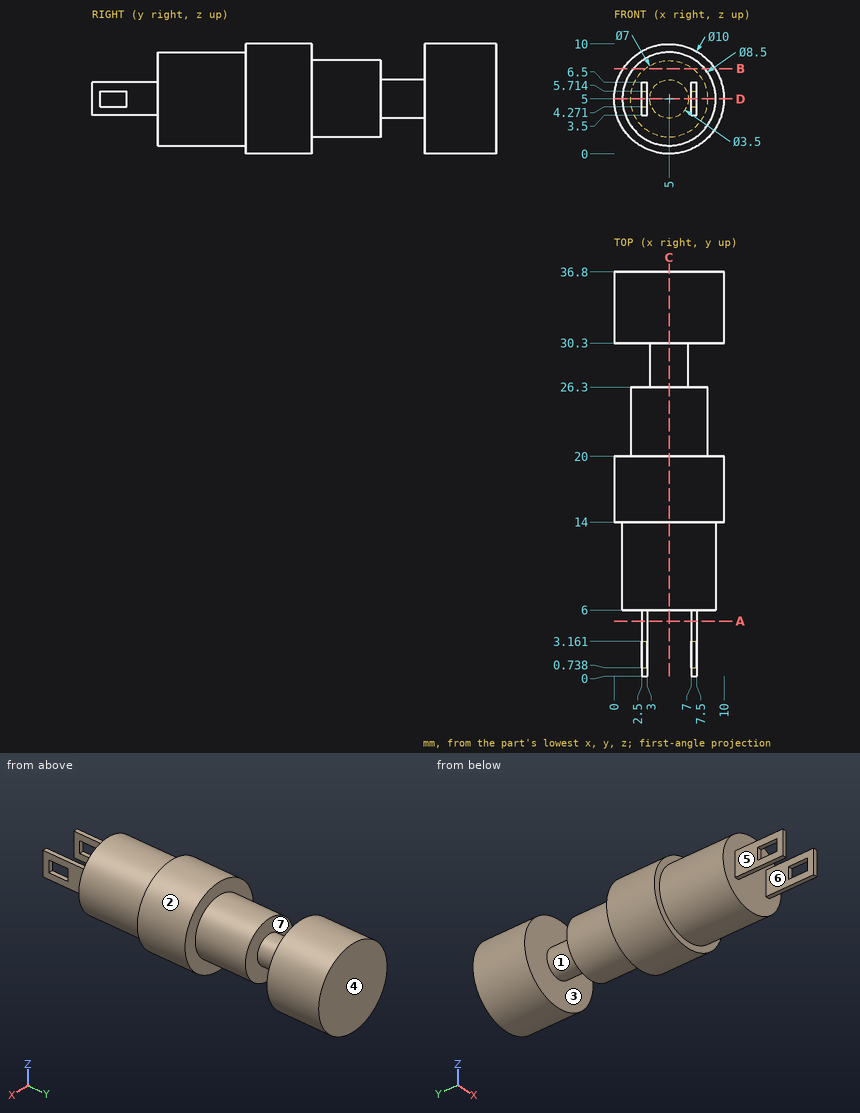
Study the drawing (mm; zero at the part's minimum x, y, z) and answer. A direction names the side the tool comes from. Give positions to 0.01 mm unless a question says otherwise; leave off trailing zeros. Order: outer loops, then holes, each group sorted by start corner. A loop starts at its lowest first (then second) coordinate and runs counter-clockwise, first axis right, second up.
1) For the marked faces 5, 6 and 7, determine the directions among +Z, -Z, +X, -X, +Y, -Y from which every point of the face is accessible in a straight line to the end or side of a thin tool.
Reported:
face 5: +Z, -Z, -X, -Y
face 6: +Z, -Z, -Y
face 7: none
2) Find section D-D on z = 5. Give the number of separate pieces and of enclosed holes in the cut face, then the cut area to 3 significant figures.
Reported:
separate pieces: 3
enclosed holes: 0
area: 255 mm2
3) Given P1, Ø3, axis at x = 6, z = 8, coming from the -Y side; P2, Ø0.9, axis at y = 2, z = 4.5, coming from the +X side; P3, Ø1, axis at x = 6, y = 19, coming from the -Z side (1 decimal), each flat-ended and moving along its own axis, determine where each tip first touches the part or whether it passes through.
Reported:
P1: stops at y = 6
P2: stops at x = 7.5
P3: stops at z = 0
4) Consider line 1 along Y through (x, z) = (5, 9); line 2 along Y through (x, z) = (6, 6.75); line 3 along Z through (x, y) = (5.25, 16). Determine where each line is inside the solid, lowest interval first.
Reported:
line 1: y = 6 to 20, 30.3 to 36.8
line 2: y = 6 to 26.3, 30.3 to 36.8
line 3: z = 0.01 to 9.99
5) Find section C-C on x = 5. Write down the section's boundary in (y, z), then the cut area to 3 significant figures.
Reported:
outline: (6, 0.75) - (14, 0.75) - (14, 0) - (20, 0) - (20, 1.5) - (26.3, 1.5) - (26.3, 3.25) - (30.3, 3.25) - (30.3, 0) - (36.8, 0) - (36.8, 10) - (30.3, 10) - (30.3, 6.75) - (26.3, 6.75) - (26.3, 8.5) - (20, 8.5) - (20, 10) - (14, 10) - (14, 9.25) - (6, 9.25) - close
area: 251 mm2
6) Find section B-B on z = 7.75. Write down the section's boundary in (x, y) (1 decimal).
Reported:
outline: (0.8, 14) - (1.8, 14) - (1.8, 6) - (8.2, 6) - (8.2, 14) - (9.2, 14) - (9.2, 20) - (7.2, 20) - (7.2, 26.3) - (2.8, 26.3) - (2.8, 20) - (0.8, 20) - close; (0.8, 30.3) - (9.2, 30.3) - (9.2, 36.8) - (0.8, 36.8) - close
7) Determine the mould class of the marked faces 1, 2, 3 and 4 for opening direction Y: pulls with the +Y half, pulls with the -Y half, needs draft (parallel to the pull), parting line crosses it, or undercut.
Reported:
face 1: undercut
face 2: needs draft
face 3: undercut
face 4: pulls with the +Y half
8) Find section A-A on y = 5. Write down the section's boundary in (x, z).
Reported:
outline: (2.5, 3.5) - (3, 3.5) - (3, 6.5) - (2.5, 6.5) - close; (7, 3.5) - (7.5, 3.5) - (7.5, 6.5) - (7, 6.5) - close
